from build123d import *

# Parameters (mm, degrees)
CUT_EXTRUDE1_DEPTH = 2
CHAMFER1_SIZE      = 0.5


with BuildPart() as part:
    # Sketch1 → Revolve1 (revolve)
    with BuildSketch(Plane.XY):
        Polygon((0, 2.5), (8, 2.5), (8, 0), (-5, 0), (-5, 4.25), (0, 4.25), align=None)
    revolve(axis=Axis((-10.4, 0, 0), (1, 0, 0)))

    # Sketch2 → Cut-Revolve1 (revolve, cut)
    with BuildSketch(Plane.XY):
        Polygon((-1.798278762, 0), (-3, 2), (-5, 2), (-5, 0), align=None)
    revolve(axis=Axis((-10.4, 0, 0), (1, 0, 0)), mode=Mode.SUBTRACT)

    # Sketch3 → Cut-Extrude1 (cut)
    with BuildSketch(Plane.ZY.offset(5)):
        Polygon((2, 1.154700538), (0, 2.309401077), (-2, 1.154700538), (-2, -1.154700538), (0, -2.309401077), (2, -1.154700538), align=None)
    extrude(amount=-CUT_EXTRUDE1_DEPTH, mode=Mode.SUBTRACT)

    # Chamfer1
    chamfer1_edges = [part.edges().sort_by_distance(p)[0] for p in [
        (-5, -4.25, 0),
        (0, -4.25, 0),
    ]]
    chamfer(chamfer1_edges, length=CHAMFER1_SIZE)


solid = part.part
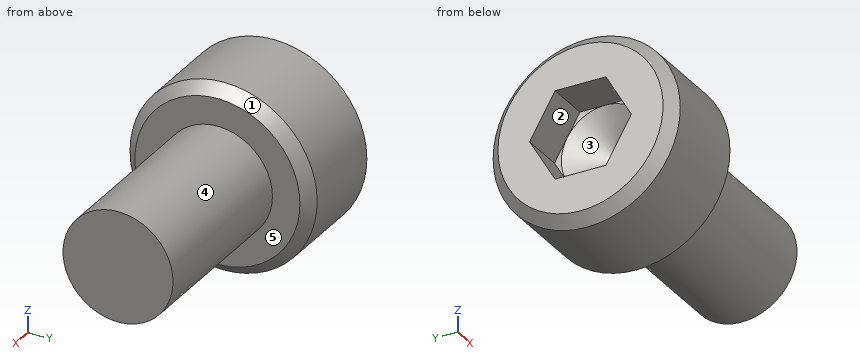
Check sheet for the modelled part. Datum: model origin and axes. Units: mm. Face numbers are marked on the shaded views. A direction names the side the tool comes from. Give positions to 0.01 mm unless a question says otherwise; leave off trailing zeros. Order: outer loops, then holes, each group sorted by start corner. A loop starts at its lowest first (then second) coordinate and runs counter-clockwise, first axis right, second up. Notation, with made-up numbers: M 24,-27 L 33,-27 A15 cw 33,-16 Z; hole C 89.25,-21.75 d4. An arc over 180 degrees is marked long. Answer as CSV lines item,"result". Start each with the question number.
Item 1: Mould release check, pull along Y, two halves, no side actions. Record for the marked faces 3, 4 and 5: +Y half, -Y half, draft (parallel to the pull), parting line (faces both ways), or undercut.
Item 2: Thickness scan on line 1 (X direction, y = -3, z = 1.25); line 2 (Z direction, x = -4.25, y = 1.5); line 3 (X direction, y = 1.75, z = -0.25). Record the ranges inside material, lowest first. Write a range as [from, to].
Item 3: Gauge pin test, flat ends, axial feed: P1, Ø3, axis at x = -1, z = 2.5, coming from the +Y side; P2, Ø2, axis at x = 4, y = -2, coming from the -Z side; P3, Ø2, axis at x = 4, z = 2, coming from the +Y side. Record the tip position at first contact, or that the pin passes through.
Item 4: Cross-section at B-B on x = -2. Enter the section's corners in (y, z), plus the area to 3 significant figures.
Item 5: Tool access check on the marked faces 1 and 2. Record the directions out of +Z, -Z, +X, -X, +Y, -Y that give a thin tool (end or side, any length) a straight path to the whole face; none if there is none.
Item 6: Cross-section at A-A on x = 0.5. Enter the section's corners in (y, z), plus the area to 3 significant figures.
Established:
1,face 3,"undercut"
1,face 4,"parting line"
1,face 5,"draft"
2,line 1,"x = [-5, 0]"
2,line 2,"z = [-3.98, -1.4], [1.4, 3.98]"
2,line 3,"x = [-2.86, 8]"
3,P1,"stops at y = 4.13"
3,P2,"stops at z = -2.29"
3,P3,"stops at y = 2.29"
4,outline,"C 0,0 d8.5; hole C 0,0 d0.67"
4,area,"56.4 mm^2"
5,face 1,"+X"
5,face 2,"-X"
6,outline,"C 0,0 d5"
6,area,"19.6 mm^2"
